Build history of the part. All positions in model axes, mm. A direction names the side the tool comes from. Give positions to 0.01 mm unless a question says otherwise; leave off trailing zeros. Write each loop counter-clockwise with the first axis right and the second up, starting at its lowest first coordinate (ties: lowest second). Pieces come first, ordered by that corner, then holes. Notation, with made-up numbers: (31.5, 53.25) -> (70.5, 53.25) arc R28 cw to (70.5, 84.25) -> close; hole circle Ø7 at (10, 17.25). An arc over 180 degrees is marked (long way). Write item = value, one per line. Start each with the question number.
Q1. Saw through at A-A, the plane z = 12.5. List the corners of the cut face in (x, y), then the cut area to 3 significant figures.
Q2. Wall check: line 1 (X direction, y = 3.6, z = -10); line 2 (X direction, y = 2.4, z = -27); line 3 (Z direction, x = 102, y = 2.6). Give the ranges that are in metal, low to high.
Q3. Tool access for faces 4 (the face through (-130, 3, 30)), 5 (the face through (-2, 0, -1)), 6 (the face through (95, 3, 30)), 7 (the face through (95, 3, -30)): list every direction of +Z, -Z, +X, -X, +Y, -Y with a clear straight run to the whole face (end or side of a thin tool).
Q4. Saw through at B-B, the plane x = -20.5. List the corners of the cut face in (y, z), then the cut area to 3 significant figures.
Q5. Saw through at C-C, the plane x = 84.5. List the corners of the cut face in (y, z), then the cut area to 3 significant figures.
Q6. Mould opens along X. For faces 1 (the face through (5, 3, 30)), 2 (the face through (-130, 3, -30)), 3 (the face through (18, 4, 0)) say: pulls with the +X half, pulls with the -X half, needs draft (parallel to the pull), parting line crosses it, or undercut.
Q7. Drop flat-ended pins along their axis: P1, Ø1.6, axis at x = 109, y = 3.5, coming from the +Z side; P2, Ø1.6, axis at y = 3, z = -10.5, coming from the +X side; P3, Ø0.6, axis at y = 3, z = -11, coming from the -X side. Give the stop position or say it passes through.
from build123d import *

# Parameters (mm, degrees)
SKETCH1_W           = 275
SKETCH1_H           = 85
BOSS_EXTRUDE1_DEPTH = 2
BOSS_EXTRUDE2_DEPTH = 2


with BuildPart() as part:
    # Sketch1 → Boss-Extrude1 (new body)
    with BuildSketch(Plane(origin=(0, 0, 0), x_dir=(1, 0, 0), z_dir=(0, 1, 0))):
        Rectangle(SKETCH1_W, SKETCH1_H)
    extrude(amount=BOSS_EXTRUDE1_DEPTH)

    # Sketch2 → Boss-Extrude2 (add)
    with BuildSketch(Plane(origin=(0, 2, 0), x_dir=(1, 0, 0), z_dir=(0, 1, 0))):
        Polygon((-100, 35), (-100, -35), (-125, -35), (-135, -25), (-135, 25), (-125, 35), align=None)
        Polygon((-90, 25), (-80, 35), (-55, 35), (-55, -35), (-80, -35), (-90, -25), align=None)
        Polygon((-45, 25), (-35, 35), (-10, 35), (-10, -35), (-35, -35), (-45, -25), align=None)
        Polygon((0, 25), (10, 35), (35, 35), (35, -35), (10, -35), (0, -25), align=None)
        Polygon((45, 25), (55, 35), (80, 35), (80, -35), (55, -35), (45, -25), align=None)
        Polygon((90, 25), (100, 35), (125, 35), (125, -35), (100, -35), (90, -25), align=None)
    extrude(amount=BOSS_EXTRUDE2_DEPTH)


solid = part.part
Report:
q1.outline = (-137.5, 0) -> (137.5, 0) -> (137.5, 2) -> (125, 2) -> (125, 4) -> (90, 4) -> (90, 2) -> (80, 2) -> (80, 4) -> (45, 4) -> (45, 2) -> (35, 2) -> (35, 4) -> (0, 4) -> (0, 2) -> (-10, 2) -> (-10, 4) -> (-45, 4) -> (-45, 2) -> (-55, 2) -> (-55, 4) -> (-90, 4) -> (-90, 2) -> (-100, 2) -> (-100, 4) -> (-135, 4) -> (-135, 2) -> (-137.5, 2) -> close
q1.area = 970 mm2
q2.line_1 = -135 to -100, -90 to -55, -45 to -10, 0 to 35, 45 to 80, 90 to 125
q2.line_2 = -133 to -100, -88 to -55, -43 to -10, 2 to 35, 47 to 80, 92 to 125
q2.line_3 = -35 to 35
q3.face_4 = +Z, -X, +Y
q3.face_5 = +Z, -Z, +X, -X, -Y
q3.face_6 = +Z, +Y
q3.face_7 = -Z, +Y
q4.outline = (0, -42.5) -> (2, -42.5) -> (2, -35) -> (4, -35) -> (4, 35) -> (2, 35) -> (2, 42.5) -> (0, 42.5) -> close
q4.area = 310 mm2
q5.outline = (0, -42.5) -> (2, -42.5) -> (2, 42.5) -> (0, 42.5) -> close
q5.area = 170 mm2
q6.face_1 = undercut
q6.face_2 = pulls with the -X half
q6.face_3 = needs draft
q7.P1 = 35
q7.P2 = 125
q7.P3 = -135
